The figure shows three views and two pictorial views of one solid part (mm, origin at its lowest corner). Answer the questions. A direction names the side the tool comes from. Coordinates: 2 decimals unless noted, no trailing zeros. Order: outer loops, then holes, each group sorted by start corner. A loop starts at its lowest first (then second) coordinate and runs counter-clockwise, first axis right, second up. Notation, with made-up numbers: (71, 1) -> (88, 1) arc R19 ccw to (88, 33) -> close; hole circle Ø9 at (42, 40). An arc over 180 degrees is marked (long way). Return JSON: item names as keys, results as strings.
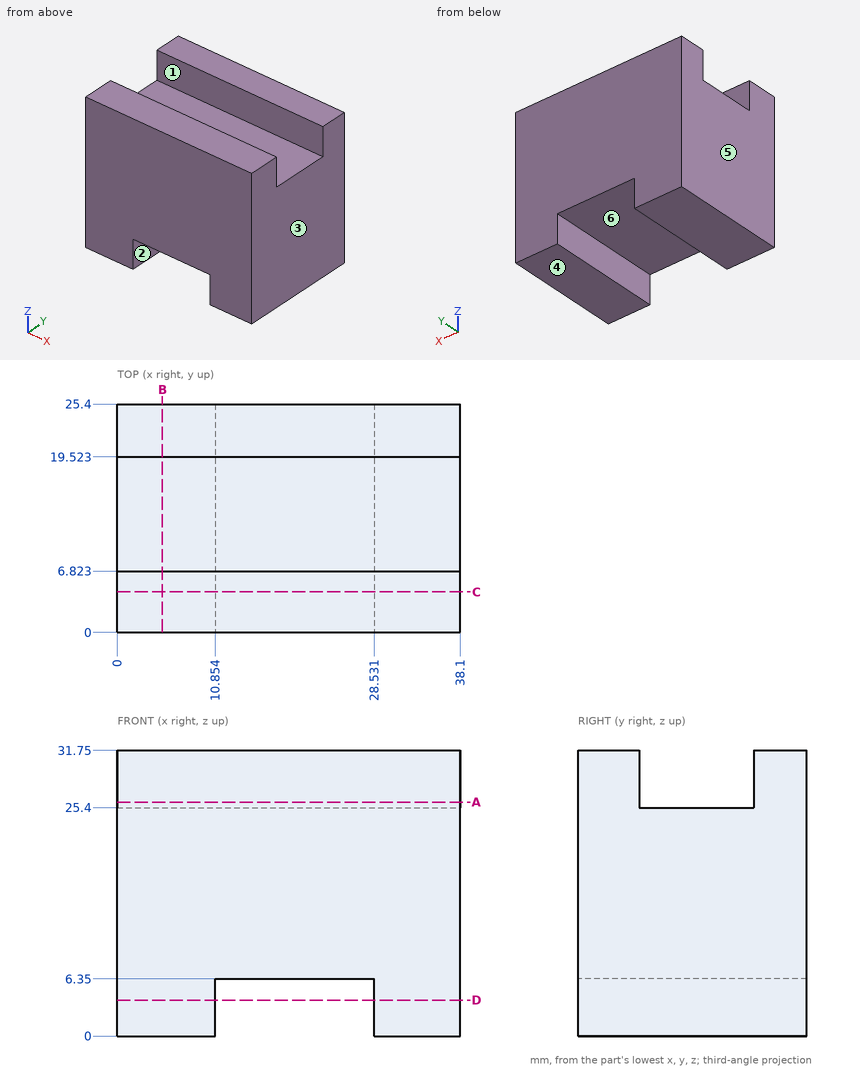
Item 1: The part is cut by section C-C on y = 4.5. Determine the outline of the cut face in (x, z).
Answer list:
{"outline": "(0, 0) -> (10.85, 0) -> (10.85, 6.35) -> (28.53, 6.35) -> (28.53, 0) -> (38.1, 0) -> (38.1, 31.75) -> (0, 31.75) -> close"}
Item 2: Determine the mould class of the marked faces 4, 5 and 6 for opening direction X: pulls with the +X half, pulls with the -X half, needs draft (parallel to the pull), parting line crosses it, or undercut.
Answer list:
{"face 4": "needs draft", "face 5": "pulls with the -X half", "face 6": "undercut"}
Item 3: The part is cut by section B-B on x = 5. Determine the outline of the cut face in (y, z).
Answer list:
{"outline": "(0, 0) -> (25.4, 0) -> (25.4, 31.75) -> (19.52, 31.75) -> (19.52, 25.4) -> (6.82, 25.4) -> (6.82, 31.75) -> (0, 31.75) -> close"}
Item 4: Which of the six approach directions +Z, -Z, +X, -X, +Y, -Y give full straight-line access (tool end or side, diameter ignored) to the marked faces 1, 2 and 3?
Answer list:
{"face 1": "+Z, +X, -X", "face 2": "-Z, +Y, -Y", "face 3": "+Z, -Z, +X, +Y, -Y"}
Item 5: Find the intervals of material crossed by probe 1 along X at (y, z) = (21, 5); probe 2 along Y at (x, z) = (9.5, 27); probe 3 along Z at (x, y) = (15.5, 9), in increasing order.
Answer list:
{"probe 1": "0 to 10.85, 28.53 to 38.1", "probe 2": "0 to 6.82, 19.52 to 25.4", "probe 3": "6.35 to 25.4"}
Item 6: The part is cut by section A-A on z = 26. Determine the outline of the cut face in (x, y).
Answer list:
{"outline": "(0, 0) -> (38.1, 0) -> (38.1, 6.82) -> (0, 6.82) -> close; (0, 19.52) -> (38.1, 19.52) -> (38.1, 25.4) -> (0, 25.4) -> close"}
Item 7: A flat-ended cylindrical pin translates along its axis: pin 1 (1 mm diameter, centred on x = 15.5, y = 22, fed in from -Z). Find the tip coordinate at first contact, or state that the pin passes through.
Answer list:
{"pin 1": "z = 6.35"}
Item 8: The part is cut by section D-D on z = 4. Determine the outline of the cut face in (x, y), plus the area to 3 significant figures.
Answer list:
{"outline": "(0, 0) -> (10.85, 0) -> (10.85, 25.4) -> (0, 25.4) -> close; (28.53, 0) -> (38.1, 0) -> (38.1, 25.4) -> (28.53, 25.4) -> close", "area": "519 mm2"}
